from build123d import *

# Parameters (mm, degrees)
SKETCH_W      = 302
SKETCH_H      = 112
SKETCH_W_2    = 287
SKETCH_H_2    = 97
PAD_DEPTH     = 4
SKETCH001_W   = 80
SKETCH001_H   = 5
SKETCH001_W_2 = 5
SKETCH001_H_2 = 32.5
POCKET_DEPTH  = 5
FILLET_R      = 1
FILLET001_R   = 1
FILLET002_R   = 1
FILLET003_R   = 1
FILLET004_R   = 1
FILLET005_R   = 1
FILLET006_R   = 1
FILLET007_R   = 1
FILLET008_R   = 1
FILLET009_R   = 1
FILLET010_R   = 1
FILLET011_R   = 1
FILLET012_R   = 1
FILLET013_R   = 1
FILLET014_R   = 1
FILLET015_R   = 1
FILLET016_R   = 1
FILLET017_R   = 1
FILLET018_R   = 1
FILLET019_R   = 1
FILLET020_R   = 1
FILLET021_R   = 1
FILLET022_R   = 1
FILLET023_R   = 1
FILLET024_R   = 1
FILLET025_R   = 1
FILLET026_R   = 1
FILLET027_R   = 1
FILLET028_R   = 1
FILLET029_R   = 1
FILLET030_R   = 1
FILLET031_R   = 1
FILLET032_R   = 1
FILLET033_R   = 1
FILLET034_R   = 1
FILLET035_R   = 1
FILLET036_R   = 1
FILLET037_R   = 1
FILLET038_R   = 1
FILLET039_R   = 1
FILLET040_R   = 1
FILLET041_R   = 1
FILLET042_R   = 1
FILLET043_R   = 1
FILLET044_R   = 1
FILLET045_R   = 1
FILLET046_R   = 1
FILLET047_R   = 1


with BuildPart() as part:
    # Sketch → Pad (new body)
    with BuildSketch(Plane.XY):
        Rectangle(SKETCH_W, SKETCH_H)
        Rectangle(SKETCH_W_2, SKETCH_H_2, mode=Mode.SUBTRACT)
    extrude(amount=PAD_DEPTH)

    # Sketch001 (on Face10 of Pad) → Pocket (cut)
    with BuildSketch(Plane.XY.offset(4)):
        with Locations((0, 51)):
            Rectangle(SKETCH001_W, SKETCH001_H)
        with Locations((0, -51)):
            Rectangle(SKETCH001_W, SKETCH001_H)
        with Locations((-95, -51)):
            Rectangle(SKETCH001_W, SKETCH001_H)
        with Locations((-95, 51)):
            Rectangle(SKETCH001_W, SKETCH001_H)
        with Locations((95, 51)):
            Rectangle(SKETCH001_W, SKETCH001_H)
        with Locations((95, -51)):
            Rectangle(SKETCH001_W, SKETCH001_H)
        with Locations((-146, 23.75)):
            Rectangle(SKETCH001_W_2, SKETCH001_H_2)
        with Locations((-146, -23.75)):
            Rectangle(SKETCH001_W_2, SKETCH001_H_2)
        with Locations((146, 23.75)):
            Rectangle(SKETCH001_W_2, SKETCH001_H_2)
        with Locations((146, -23.75)):
            Rectangle(SKETCH001_W_2, SKETCH001_H_2)
    extrude(amount=-POCKET_DEPTH, mode=Mode.SUBTRACT)

    # Fillet
    fillet_edges = [part.edges().sort_by_distance(p)[0] for p in [
        (-151, -56, 2),
    ]]
    fillet(fillet_edges, radius=FILLET_R)

    # Fillet001
    fillet001_edges = [part.edges().sort_by_distance(p)[0] for p in [
        (-143.5, -7.5, 2),
    ]]
    fillet(fillet001_edges, radius=FILLET001_R)

    # Fillet002
    fillet002_edges = [part.edges().sort_by_distance(p)[0] for p in [
        (-55, -48.5, 2),
    ]]
    fillet(fillet002_edges, radius=FILLET002_R)

    # Fillet003
    fillet003_edges = [part.edges().sort_by_distance(p)[0] for p in [
        (40, -48.5, 2),
    ]]
    fillet(fillet003_edges, radius=FILLET003_R)

    # Fillet004
    fillet004_edges = [part.edges().sort_by_distance(p)[0] for p in [
        (135, -48.5, 2),
    ]]
    fillet(fillet004_edges, radius=FILLET004_R)

    # Fillet005
    fillet005_edges = [part.edges().sort_by_distance(p)[0] for p in [
        (143.5, -40, 2),
    ]]
    fillet(fillet005_edges, radius=FILLET005_R)

    # Fillet006
    fillet006_edges = [part.edges().sort_by_distance(p)[0] for p in [
        (151, -56, 2),
    ]]
    fillet(fillet006_edges, radius=FILLET006_R)

    # Fillet007
    fillet007_edges = [part.edges().sort_by_distance(p)[0] for p in [
        (148.5, -7.5, 2),
    ]]
    fillet(fillet007_edges, radius=FILLET007_R)

    # Fillet008
    fillet008_edges = [part.edges().sort_by_distance(p)[0] for p in [
        (143.5, -7.5, 2),
    ]]
    fillet(fillet008_edges, radius=FILLET008_R)

    # Fillet009
    fillet009_edges = [part.edges().sort_by_distance(p)[0] for p in [
        (143.5, 7.5, 2),
    ]]
    fillet(fillet009_edges, radius=FILLET009_R)

    # Fillet010
    fillet010_edges = [part.edges().sort_by_distance(p)[0] for p in [
        (148.5, 40, 2),
    ]]
    fillet(fillet010_edges, radius=FILLET010_R)

    # Fillet011
    fillet011_edges = [part.edges().sort_by_distance(p)[0] for p in [
        (143.5, 40, 2),
    ]]
    fillet(fillet011_edges, radius=FILLET011_R)

    # Fillet012
    fillet012_edges = [part.edges().sort_by_distance(p)[0] for p in [
        (143.5, 48.5, 2),
    ]]
    fillet(fillet012_edges, radius=FILLET012_R)

    # Fillet013
    fillet013_edges = [part.edges().sort_by_distance(p)[0] for p in [
        (135, 48.5, 2),
    ]]
    fillet(fillet013_edges, radius=FILLET013_R)

    # Fillet014
    fillet014_edges = [part.edges().sort_by_distance(p)[0] for p in [
        (135, 53.5, 2),
    ]]
    fillet(fillet014_edges, radius=FILLET014_R)

    # Fillet015
    fillet015_edges = [part.edges().sort_by_distance(p)[0] for p in [
        (55, 48.5, 2),
    ]]
    fillet(fillet015_edges, radius=FILLET015_R)

    # Fillet016
    fillet016_edges = [part.edges().sort_by_distance(p)[0] for p in [
        (40, 48.5, 2),
    ]]
    fillet(fillet016_edges, radius=FILLET016_R)

    # Fillet017
    fillet017_edges = [part.edges().sort_by_distance(p)[0] for p in [
        (40, 53.5, 2),
    ]]
    fillet(fillet017_edges, radius=FILLET017_R)

    # Fillet018
    fillet018_edges = [part.edges().sort_by_distance(p)[0] for p in [
        (-40, 48.5, 2),
    ]]
    fillet(fillet018_edges, radius=FILLET018_R)

    # Fillet019
    fillet019_edges = [part.edges().sort_by_distance(p)[0] for p in [
        (-55, 48.5, 2),
    ]]
    fillet(fillet019_edges, radius=FILLET019_R)

    # Fillet020
    fillet020_edges = [part.edges().sort_by_distance(p)[0] for p in [
        (-55, 53.5, 2),
    ]]
    fillet(fillet020_edges, radius=FILLET020_R)

    # Fillet021
    fillet021_edges = [part.edges().sort_by_distance(p)[0] for p in [
        (-143.5, 40, 2),
    ]]
    fillet(fillet021_edges, radius=FILLET021_R)

    # Fillet022
    fillet022_edges = [part.edges().sort_by_distance(p)[0] for p in [
        (-135, 48.5, 2),
    ]]
    fillet(fillet022_edges, radius=FILLET022_R)

    # Fillet023
    fillet023_edges = [part.edges().sort_by_distance(p)[0] for p in [
        (-151, 56, 2),
    ]]
    fillet(fillet023_edges, radius=FILLET023_R)

    # Fillet024
    fillet024_edges = [part.edges().sort_by_distance(p)[0] for p in [
        (-143.5, 48.5, 2),
    ]]
    fillet(fillet024_edges, radius=FILLET024_R)

    # Fillet025
    fillet025_edges = [part.edges().sort_by_distance(p)[0] for p in [
        (-135, 53.5, 2),
    ]]
    fillet(fillet025_edges, radius=FILLET025_R)

    # Fillet026
    fillet026_edges = [part.edges().sort_by_distance(p)[0] for p in [
        (-148.5, 40, 2),
    ]]
    fillet(fillet026_edges, radius=FILLET026_R)

    # Fillet027
    fillet027_edges = [part.edges().sort_by_distance(p)[0] for p in [
        (-148.5, -7.5, 2),
    ]]
    fillet(fillet027_edges, radius=FILLET027_R)

    # Fillet028
    fillet028_edges = [part.edges().sort_by_distance(p)[0] for p in [
        (-143.5, -40, 2),
    ]]
    fillet(fillet028_edges, radius=FILLET028_R)

    # Fillet029
    fillet029_edges = [part.edges().sort_by_distance(p)[0] for p in [
        (-135, -48.5, 2),
    ]]
    fillet(fillet029_edges, radius=FILLET029_R)

    # Fillet030
    fillet030_edges = [part.edges().sort_by_distance(p)[0] for p in [
        (55, 53.5, 2),
    ]]
    fillet(fillet030_edges, radius=FILLET030_R)

    # Fillet031
    fillet031_edges = [part.edges().sort_by_distance(p)[0] for p in [
        (-40, 53.5, 2),
    ]]
    fillet(fillet031_edges, radius=FILLET031_R)

    # Fillet032
    fillet032_edges = [part.edges().sort_by_distance(p)[0] for p in [
        (-148.5, 7.5, 2),
    ]]
    fillet(fillet032_edges, radius=FILLET032_R)

    # Fillet033
    fillet033_edges = [part.edges().sort_by_distance(p)[0] for p in [
        (-143.5, 7.5, 2),
    ]]
    fillet(fillet033_edges, radius=FILLET033_R)

    # Fillet034
    fillet034_edges = [part.edges().sort_by_distance(p)[0] for p in [
        (-148.5, -40, 2),
    ]]
    fillet(fillet034_edges, radius=FILLET034_R)

    # Fillet035
    fillet035_edges = [part.edges().sort_by_distance(p)[0] for p in [
        (-143.5, -48.5, 2),
    ]]
    fillet(fillet035_edges, radius=FILLET035_R)

    # Fillet036
    fillet036_edges = [part.edges().sort_by_distance(p)[0] for p in [
        (-135, -53.5, 2),
    ]]
    fillet(fillet036_edges, radius=FILLET036_R)

    # Fillet037
    fillet037_edges = [part.edges().sort_by_distance(p)[0] for p in [
        (-40, -48.5, 2),
    ]]
    fillet(fillet037_edges, radius=FILLET037_R)

    # Fillet038
    fillet038_edges = [part.edges().sort_by_distance(p)[0] for p in [
        (-40, -53.5, 2),
    ]]
    fillet(fillet038_edges, radius=FILLET038_R)

    # Fillet039
    fillet039_edges = [part.edges().sort_by_distance(p)[0] for p in [
        (55, -48.5, 2),
    ]]
    fillet(fillet039_edges, radius=FILLET039_R)

    # Fillet040
    fillet040_edges = [part.edges().sort_by_distance(p)[0] for p in [
        (55, -53.5, 2),
    ]]
    fillet(fillet040_edges, radius=FILLET040_R)

    # Fillet041
    fillet041_edges = [part.edges().sort_by_distance(p)[0] for p in [
        (-55, -53.5, 2),
    ]]
    fillet(fillet041_edges, radius=FILLET041_R)

    # Fillet042
    fillet042_edges = [part.edges().sort_by_distance(p)[0] for p in [
        (40, -53.5, 2),
    ]]
    fillet(fillet042_edges, radius=FILLET042_R)

    # Fillet043
    fillet043_edges = [part.edges().sort_by_distance(p)[0] for p in [
        (151, 56, 2),
    ]]
    fillet(fillet043_edges, radius=FILLET043_R)

    # Fillet044
    fillet044_edges = [part.edges().sort_by_distance(p)[0] for p in [
        (143.5, -48.5, 2),
    ]]
    fillet(fillet044_edges, radius=FILLET044_R)

    # Fillet045
    fillet045_edges = [part.edges().sort_by_distance(p)[0] for p in [
        (135, -53.5, 2),
    ]]
    fillet(fillet045_edges, radius=FILLET045_R)

    # Fillet046
    fillet046_edges = [part.edges().sort_by_distance(p)[0] for p in [
        (148.5, -40, 2),
    ]]
    fillet(fillet046_edges, radius=FILLET046_R)

    # Fillet047
    fillet047_edges = [part.edges().sort_by_distance(p)[0] for p in [
        (148.5, 7.5, 2),
    ]]
    fillet(fillet047_edges, radius=FILLET047_R)


solid = part.part
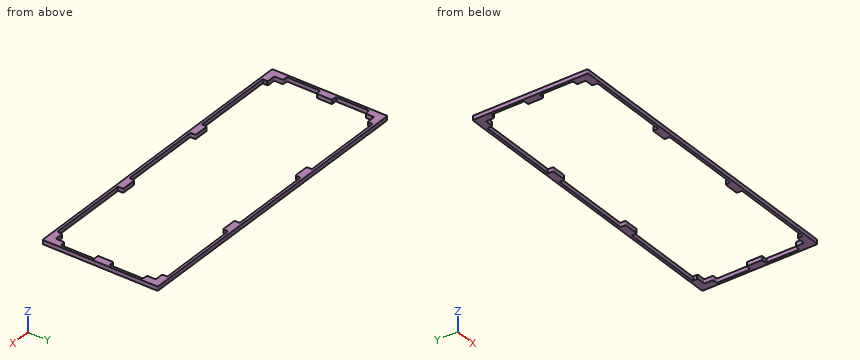
Could you check a few things on this model? Use its own coordinates, in mm. Round coordinates to 2 decimals unless told otherwise and drop trailing zeros. Loops run counter-clockwise (first coordinate to the right, second up) from the corner with the lowest first, then second, coordinate; pieces in that order, holes last. Notation, with made-up numbers: (-12, 2) - (-7, 2) arc R14 ccw to (-7, 26) - close; hole circle Ø8 at (-12, 57). An arc over 180 degrees is marked (long way). Write item = value, one per line.
1) Imagine slicing it at B-B (x = 127.5). Please give me the cut outline in (y, z).
Computed:
outline = (-56, 0) - (-53.5, 0) - (-53.5, 4) - (-56, 4) - close; (53.5, 0) - (56, 0) - (56, 4) - (53.5, 4) - close
2) I need wall thicknesses on line 1 along X through (y, z) = (-50.5, 0.35); line 2 along Y through (x, z) = (-117, 3.85); line 3 along X through (y, z) = (20, 2). Which ranges of each line are inside material? Lowest first, please. Write a range as from..to.
Computed:
line_1 = -151..-135, -55..-40, 40..55, 135..151
line_2 = -56..-53.5, 53.5..56
line_3 = -151..-148.5, 148.5..151
3) Imagine slicing it at A-A (y = 34.5). Please give me the cut outline in (x, z).
Computed:
outline = (-151, 0) - (-148.5, 0) - (-148.5, 4) - (-151, 4) - close; (148.5, 0) - (151, 0) - (151, 4) - (148.5, 4) - close
